For this review, take the finished solid that the model builds, in its own axes (mm). Coordinates: 2 decimals unless noted, no trailing zeros. Loops run counter-clockwise (first coordinate to the right, second up) from the corner with the lowest first, then second, coordinate; pieces in that order, holes last. Notation, with made-up numbers: (-22, 83.25) - (-12, 83.25) arc R22 cw to (-12, 121.25) - close; hole circle Ø9 at (45.5, 62.25). An arc over 180 degrees is marked (long way). One line per item, written item: value. Start each with the question number.
1. Insertion check: pin 1 (1.5 mm diameter, centred on x = -18, y = 37, fed in from +Z); pin 2 (2 mm diameter, centred on y = 179.5, z = -2, fed in from -X); pin 3 (3 mm diameter, centred on y = 202.5, z = -3.5, fed in from -X); pin 4 (2 mm diameter, centred on y = 188.5, z = -3.5, fed in from -X). Each pin has a flat end and moves straight along its axis. Give the tip position at first contact, or say it passes through.
2. Take a section at C-C, the plane x = -21. State the section outline as (y, z) points.
3. Take a section at B-B, the plane y = 166.5. State the section outline as (x, z) points.
4. To check wall thickness, follow line 1 (Y direction, x = 52, z = -3.4); line 2 (Y direction, x = 97, z = -0.85); line 3 (Y direction, x = 139.5, z = -3.6). State the ranges of each line that lie inside material, in increasing order. Write a range as from..to.
5. Take a section at A-A, the plane z = -3.25. Count the separate pieces of the cut face and the enclosed holes in it, and give its area (3 significant figures).
```python
from build123d import *

# Parameters (mm, degrees)
SKETCH1_R           = 1.5
SKETCH1_W           = 8
SKETCH1_H           = 8
SKETCH1_W_2         = 25
SKETCH1_H_2         = 4
SKETCH1_W_3         = 18
BOSS_EXTRUDE3_DEPTH = 6
SKETCH1_9_R         = 1.5
CUT_EXTRUDE2_DEPTH  = 6


with BuildPart() as part:
    # Sketch1 → Boss-Extrude3 (new body)
    with BuildSketch(Plane.XY):
        with BuildLine():
            Line((-36.07279856, -10.151608153), (153.92720144, -10.151608153))
            ThreePointArc((153.92720144, -10.151608153), (160.998269252, -7.222675965), (163.92720144, -0.151608153))
            Line((163.92720144, -0.151608153), (163.92720144, 59.848391847))
            ThreePointArc((163.92720144, 59.848391847), (160.998269252, 66.919459659), (153.92720144, 69.848391847))
            Line((153.92720144, 69.848391847), (108.92720144, 69.848391847))
            ThreePointArc((108.92720144, 69.848391847), (105.391667534, 71.312857941), (103.92720144, 74.848391847))
            Line((103.92720144, 74.848391847), (103.92720144, 84.848391847))
            ThreePointArc((103.92720144, 84.848391847), (102.462735346, 88.383925753), (98.92720144, 89.848391847))
            Line((98.92720144, 89.848391847), (78.92720144, 89.848391847))
            Line((78.92720144, 89.848391847), (68.638210005, 154.848391847))
            Line((68.638210005, 154.848391847), (81.638210005, 154.848391847))
            Line((81.638210005, 154.848391847), (81.638210005, 174.848391847))
            ThreePointArc((81.638210005, 174.848391847), (83.102676099, 178.383925753), (86.638210005, 179.848391847))
            Line((86.638210005, 179.848391847), (121.92720144, 179.848391847))
            ThreePointArc((121.92720144, 179.848391847), (123.341415002, 180.434178284), (123.92720144, 181.848391847))
            Line((123.92720144, 181.848391847), (123.92720144, 193.848391847))
            ThreePointArc((123.92720144, 193.848391847), (123.341415002, 195.262605409), (121.92720144, 195.848391847))
            Line((121.92720144, 195.848391847), (81.92720144, 195.848391847))
            ThreePointArc((81.92720144, 195.848391847), (80.512987878, 196.434178284), (79.92720144, 197.848391847))
            Line((79.92720144, 197.848391847), (79.92720144, 210))
            ThreePointArc((79.92720144, 210), (78.755628565, 212.828427125), (75.92720144, 214))
            Line((75.92720144, 214), (41.92720144, 214))
            ThreePointArc((41.92720144, 214), (39.098774315, 212.828427125), (37.92720144, 210))
            Line((37.92720144, 210), (37.92720144, 197.848391847))
            ThreePointArc((37.92720144, 197.848391847), (37.341415002, 196.434178284), (35.92720144, 195.848391847))
            Line((35.92720144, 195.848391847), (-4.07279856, 195.848391847))
            ThreePointArc((-4.07279856, 195.848391847), (-5.487012122, 195.262605409), (-6.07279856, 193.848391847))
            Line((-6.07279856, 193.848391847), (-6.07279856, 181.848391847))
            ThreePointArc((-6.07279856, 181.848391847), (-5.487012122, 180.434178284), (-4.07279856, 179.848391847))
            Line((-4.07279856, 179.848391847), (30.638210005, 179.848391847))
            ThreePointArc((30.638210005, 179.848391847), (34.173743911, 178.383925753), (35.638210005, 174.848391847))
            Line((35.638210005, 174.848391847), (35.638210005, 154.848391847))
            Line((35.638210005, 154.848391847), (48.638210005, 154.848391847))
            Line((48.638210005, 154.848391847), (38.92720144, 89.848391847))
            Line((38.92720144, 89.848391847), (18.92720144, 89.848391847))
            ThreePointArc((18.92720144, 89.848391847), (15.391667534, 88.383925753), (13.92720144, 84.848391847))
            Line((13.92720144, 84.848391847), (13.92720144, 74.848391847))
            ThreePointArc((13.92720144, 74.848391847), (12.462735346, 71.312857941), (8.92720144, 69.848391847))
            Line((8.92720144, 69.848391847), (-36.07279856, 69.848391847))
            ThreePointArc((-36.07279856, 69.848391847), (-43.143866372, 66.919459659), (-46.07279856, 59.848391847))
            Line((-46.07279856, 59.848391847), (-46.07279856, -0.151608153))
            ThreePointArc((-46.07279856, -0.151608153), (-43.143866372, -7.222675965), (-36.07279856, -10.151608153))
        make_face()
        with Locations((143.638210005, 57.5)):
            Circle(SKETCH1_R, mode=Mode.SUBTRACT)
        with Locations((132.413840271, 57.5)):
            Circle(SKETCH1_R, mode=Mode.SUBTRACT)
        with Locations((132.413840271, 12.5)):
            Circle(SKETCH1_R, mode=Mode.SUBTRACT)
        with Locations((143.638210005, 12.5)):
            Circle(SKETCH1_R, mode=Mode.SUBTRACT)
        with Locations((117.638210005, 182.5)):
            Circle(SKETCH1_R, mode=Mode.SUBTRACT)
        with Locations((117.638210005, 192.5)):
            Circle(SKETCH1_R, mode=Mode.SUBTRACT)
        with Locations((-0.361789995, 182.5)):
            Circle(SKETCH1_R, mode=Mode.SUBTRACT)
        with Locations((-0.361789995, 192.5)):
            Circle(SKETCH1_R, mode=Mode.SUBTRACT)
        with Locations((26.638210005, 182.5)):
            Circle(SKETCH1_R, mode=Mode.SUBTRACT)
        with Locations((90.638210005, 182.5)):
            Circle(SKETCH1_R, mode=Mode.SUBTRACT)
        with Locations((92.638210005, 189)):
            Rectangle(SKETCH1_W, SKETCH1_H, mode=Mode.SUBTRACT)
        with Locations((58.638210005, 188)):
            Rectangle(SKETCH1_W_2, SKETCH1_H_2, mode=Mode.SUBTRACT)
        with Locations((58.638210005, 207)):
            Rectangle(SKETCH1_W_3, SKETCH1_H_2, mode=Mode.SUBTRACT)
    extrude(amount=-BOSS_EXTRUDE3_DEPTH)

    # Sketch1<9> → Cut-Extrude2 (cut)
    with BuildSketch(Plane.XY):
        with Locations((98.92720144, 84.848391847)):
            Circle(SKETCH1_9_R)
        with Locations((18.92720144, 84.848391847)):
            Circle(SKETCH1_9_R)
        with Locations((98.92720144, 4.848391847)):
            Circle(SKETCH1_9_R)
        with Locations((18.92720144, 4.848391847)):
            Circle(SKETCH1_9_R)
    extrude(amount=-CUT_EXTRUDE2_DEPTH, mode=Mode.SUBTRACT)


solid = part.part
```
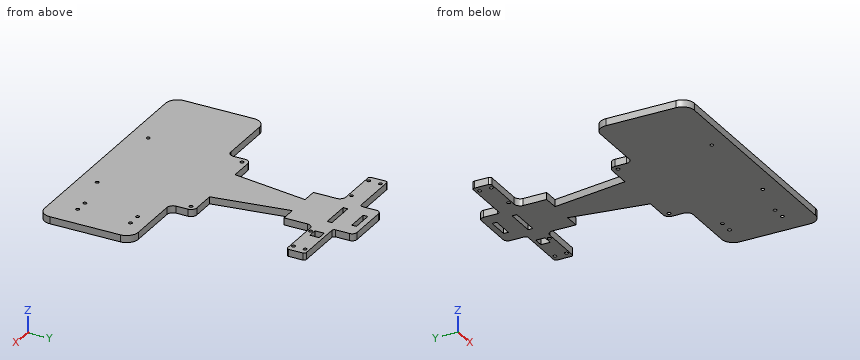
Solutions:
1. pin 1: z = 0
1. pin 2: x = -5.55
1. pin 3: x = 37.93
1. pin 4: x = -6.07
2. outline: (-10.15, -6) - (69.85, -6) - (69.85, 0) - (-10.15, 0) - close
3. outline: (35.64, -6) - (81.64, -6) - (81.64, 0) - (35.64, 0) - close
4. line 1: -10.15..186, 190..205, 209..214
4. line 2: -10.15..89.85, 179.85..195.85
4. line 3: -10.15..69.85
5. separate pieces: 1
5. enclosed holes: 17
5. area: 24,100 mm2
